from build123d import *

# Parameters (mm, degrees)
F_01_LINK_PROFILE_W            = 660
F_01_LINK_PROFILE_H            = 150
F_01_LINK_PROFILE_R            = 52.5
F_01_LINK_PROFILE_W_2          = 330
F_01_LINK_PROFILE_H_2          = 58
F_01_LINK_PLATE_DEPTH          = 22
F_02_END_BOSS_PROFILES_R       = 69
F_02_END_BOSS_PROFILES_R_2     = 52.5
F_02_BEARING_SEAT_BOSSES_DEPTH = 38
F_03_CENTER_RIB_PROFILE_W      = 360
F_03_CENTER_RIB_PROFILE_H      = 24
F_03_CENTER_RIB_DEPTH          = 34


with BuildPart() as part:
    # 01_Link_Profile → 01_Link_Plate (new body)
    with BuildSketch(Plane(origin=(0, 0, 0), x_dir=(1, 0, 0), z_dir=(0, 1, 0))):
        Rectangle(F_01_LINK_PROFILE_W, F_01_LINK_PROFILE_H)
        with Locations(Location((-272.5, 0, 0), (0, 0, 270))):
            Circle(F_01_LINK_PROFILE_R, mode=Mode.SUBTRACT)
        with Locations(Location((272.5, 0, 0), (0, 0, 270))):
            Circle(F_01_LINK_PROFILE_R, mode=Mode.SUBTRACT)
        Rectangle(F_01_LINK_PROFILE_W_2, F_01_LINK_PROFILE_H_2, mode=Mode.SUBTRACT)
    extrude(amount=F_01_LINK_PLATE_DEPTH)

    # 02_End_Boss_Profiles → 02_Bearing_Seat_Bosses (add)
    # profile 1 of 2: a face of its own
    with BuildSketch(Plane(origin=(0, 0, 0), x_dir=(1, 0, 0), z_dir=(0, 1, 0))):
        with Locations(Location((-272.5, 0, 0), (0, 0, 146.442690238))):
            Circle(F_02_END_BOSS_PROFILES_R)
        with Locations(Location((-272.5, 0, 0), (0, 0, 270))):
            Circle(F_02_END_BOSS_PROFILES_R_2, mode=Mode.SUBTRACT)
    # profile 2 of 2: a face of its own
    with BuildSketch(Plane(origin=(0, 0, 0), x_dir=(1, 0, 0), z_dir=(0, 1, 0))):
        with Locations(Location((272.5, 0, 0), (0, 0, 33.557309762))):
            Circle(F_02_END_BOSS_PROFILES_R)
        with Locations(Location((272.5, 0, 0), (0, 0, 270))):
            Circle(F_02_END_BOSS_PROFILES_R_2, mode=Mode.SUBTRACT)
    extrude(amount=F_02_BEARING_SEAT_BOSSES_DEPTH)

    # 03_Center_Rib_Profile → 03_Center_Rib (add)
    with BuildSketch(Plane(origin=(0, 0, 0), x_dir=(1, 0, 0), z_dir=(0, 1, 0))):
        Rectangle(F_03_CENTER_RIB_PROFILE_W, F_03_CENTER_RIB_PROFILE_H)
    extrude(amount=F_03_CENTER_RIB_DEPTH)


solid = part.part
Part model, mm, in its own coordinate system. A direction names the side the tool comes from. Coordinates: 2 decimals unless noted, no trailing zeros. Loops run counter-clockwise (first coordinate to the right, second up) from the corner with the lowest first, then second, coordinate; pieces in that order, holes last. Notation, with made-up numbers: M 72.25,77 L 96.25,77 A22 cw 96.25,104 Z; hole C 82,17 d6. An arc over 180 degrees is marked long. Use a Markdown table: item, result. Add a question column.
Q1. Pin check, flat tips, straight feed: P1, Ø17.5, axis at y = 6, z = 57, coming from the +X side; P2, Ø12, axis at x = 9, z = 4.5, coming from the +Y side; P3, Ø6, axis at y = 28, z = -2.5, coming from the +X side. Stop position of each tip, or through.
Q2. Cut at C-C (y = 11). Write the cut outline in (x, z).
Q3. Cut at D-D (x = -272.5). Write the cut outline in (y, z).
Q4. Probe L1, parallel to Z at x = -152.5, y = 15; L2, parallel to X at y = 29, z = 0; L3, parallel to X at y = 14, z = 0. List the from-to ranges inside material, lowest first.
Q5. Cut at B-B (z = 0). Write the cut outline in (x, y), and give its area (3 significant figures).
Q6. Mould opens along X. For faces 1 (the flat face through (330, 11, -56)), 2 (the flat face through (-180, 28, 0)), 3 (the flat face through (-292, 38, 49)) say: +X half, -X half, draft (parallel to the pull), parting line (faces both ways), or undercut.
Q7. Cut at A-A (x = 157). Write the cut outline in (y, z), and give its area (3 significant figures).
Q8. Which spindle directions (+Z, -Z, +X, -X, +Y, -Y) get a long thin tool onto all of the face, cutting with end or side? Do faces 4 (the flat face through (165, 11, 21)), 5 (the flat face through (-330, 11, -56)), 6 (the flat face through (-5, 22, -34)), 7 (the flat face through (330, 11, 57)). Say none if no direction does.
Worked out:
| question | item | result |
|---|---|---|
| 1 | P1 | stops at x = 330 |
| 1 | P2 | stops at y = 34 |
| 1 | P3 | stops at x = 341.5 |
| 2 | outline | M -330,-75 L 330,-75 L 330,-38.14 A69 ccw 330,38.14 L 330,75 L -330,75 L -330,38.14 A69 ccw -330,-38.14 Z; hole C -272.5,0 d105; hole M -165,-29 L 165,-29 L 165,-12 L -165,-12 Z; hole M -165,12 L 165,12 L 165,29 L -165,29 Z; hole C 272.5,0 d105 |
| 3 | outline | M 0,-75 L 22,-75 L 22,-69 L 38,-69 L 38,-52.5 L 0,-52.5 Z; M 0,52.5 L 38,52.5 L 38,69 L 22,69 L 22,75 L 0,75 Z |
| 4 | L1 | z = -75 to -29, -12 to 12, 29 to 75 |
| 4 | L2 | x = -341.5 to -325, -220 to -203.5, -180 to 180, 203.5 to 220, 325 to 341.5 |
| 4 | L3 | x = -341.5 to -325, -220 to 220, 325 to 341.5 |
| 5 | outline | M -341.5,0 L -325,0 L -325,38 L -341.5,38 Z; M -220,0 L 220,0 L 220,38 L 203.5,38 L 203.5,22 L 180,22 L 180,34 L -180,34 L -180,22 L -203.5,22 L -203.5,38 L -220,38 Z; M 325,0 L 341.5,0 L 341.5,38 L 325,38 Z |
| 5 | area | 15,800 mm2 |
| 6 | face 1 | +X half |
| 6 | face 2 | undercut |
| 6 | face 3 | draft |
| 7 | outline | M 0,-75 L 22,-75 L 22,-29 L 0,-29 Z; M 0,-12 L 34,-12 L 34,12 L 0,12 Z; M 0,29 L 22,29 L 22,75 L 0,75 Z |
| 7 | area | 2,840 mm2 |
| 8 | face 4 | +Y, -Y |
| 8 | face 5 | -Z, -X, +Y, -Y |
| 8 | face 6 | +Y |
| 8 | face 7 | +Z, +X, +Y, -Y |
